```python
from build123d import *

# Parameters (mm, degrees)
BOSS_EXTRUDE1_DEPTH     = 16
SKETCH8_R               = 3.5
CUT_EXTRUDE1_DEPTH      = 16
SKETCH11_R              = 3.5
CUT_EXTRUDE2_DEPTH      = 16
CUT_EXTRUDE3_DEPTH      = 56.172456897
CUT_EXTRUDE3_DEPTH_BACK = 56.172456897
SKETCH12_R              = 3.5
CUT_EXTRUDE4_DEPTH      = 63.497999968
CUT_EXTRUDE4_DEPTH_BACK = 63.497999968
CUT_EXTRUDE5_DEPTH      = 63.497999968
CUT_EXTRUDE5_DEPTH_BACK = 63.497999968


with BuildPart() as part:
    # Sketch3 → Boss-Extrude1 (new body)
    with BuildSketch(Plane.XY):
        Polygon((0, 0), (21, 0), (21, 10), (34, 10), (34, 0), (55, 0), (55, 7), (42, 7), (42, 32), (32, 32), (32, 17), (23, 17), (23, 32), (13, 32), (13, 7), (0, 7), align=None)
    extrude(amount=BOSS_EXTRUDE1_DEPTH)

    # Sketch8 → Cut-Extrude1 (cut)
    with BuildSketch(Plane(origin=(0, 7, 0), x_dir=(1, 0, 0), z_dir=(0, 1, 0))):
        with Locations(Location((6.5, -8, 0), (0, 0, 270))):
            Circle(SKETCH8_R)
    extrude(amount=-CUT_EXTRUDE1_DEPTH, mode=Mode.SUBTRACT)

    # Sketch11 → Cut-Extrude2 (cut)
    with BuildSketch(Plane(origin=(0, 7, 0), x_dir=(1, 0, 0), z_dir=(0, 1, 0))):
        with Locations(Location((48.5, -8, 0), (0, 0, 270))):
            Circle(SKETCH11_R)
    extrude(amount=-CUT_EXTRUDE2_DEPTH, mode=Mode.SUBTRACT)

    # Sketch12 → Cut-Extrude3 (cut, two sides: drawn at the far end of the back side and taken through both)
    with BuildSketch(Plane.ZY.offset(-13).offset(-CUT_EXTRUDE3_DEPTH_BACK)):
        with Locations((8, 24)):
            Circle(SKETCH12_R)
    extrude(amount=CUT_EXTRUDE3_DEPTH + CUT_EXTRUDE3_DEPTH_BACK, mode=Mode.SUBTRACT)

    # Sketch13 → Cut-Extrude4 (cut, two sides: drawn at the far end of the back side and taken through both)
    with BuildSketch(Plane(origin=(0, 7, 0), x_dir=(1, 0, 0), z_dir=(0, 1, 0)).offset(-CUT_EXTRUDE4_DEPTH_BACK)):
        Polygon((6.5, -16), (0, -16), (0, -10), align=None)
    extrude(amount=CUT_EXTRUDE4_DEPTH + CUT_EXTRUDE4_DEPTH_BACK, mode=Mode.SUBTRACT)

    # Sketch14 → Cut-Extrude5 (cut, two sides: drawn at the far end of the back side and taken through both)
    with BuildSketch(Plane(origin=(0, 7, 0), x_dir=(1, 0, 0), z_dir=(0, 1, 0)).offset(-CUT_EXTRUDE5_DEPTH_BACK)):
        Polygon((55, -16), (55, -10), (48.5, -16), align=None)
    extrude(amount=CUT_EXTRUDE5_DEPTH + CUT_EXTRUDE5_DEPTH_BACK, mode=Mode.SUBTRACT)


solid = part.part
```
Can you work these out from the model? Positions are in its coordinate system, mm. A direction names the side the tool comes from. Coordinates: 2 decimals unless noted, no trailing zeros. Order: outer loops, then holes, each group sorted by start corner. A loop starts at its lowest first (then second) coordinate and runs counter-clockwise, first axis right, second up.
1. If we section it at C-C (x = 46): Please give me the cut outline in (y, z).
2. If we section it at D-D (z = 1.25): Please give me the cut outline in (x, y), then the cut area to 3 significant figures.
3. I need wall thicknesses on line 1 (X direction, y = 2, z = 8); line 2 (X direction, y = 19, z = 3.75); line 3 (Y direction, x = 36.25, z = 8). Which ranges of each line are inside material? Lowest first, please.
4. Thinking about a two-plate mould opening in X: for faces 1 (the face through (21, 5, 8)), 2 (the face through (10.4, 0, 7.9)), 3 (the face through (42, 19, 8)), which applies, +X half, -X half, draft (parallel to the pull), parting line (faces both ways), or undercut?
5. If we section it at A-A (z = 8): Give the number of separate pieces and of enclosed holes in the cut face, then the cut area to 3 significant figures.
6. I'm going to push flat-ended pins straight in: pin 1 (5 mm diameter, centred on y = 22.5, z = 4.5, fed in from +X); pin 2 (4 mm diameter, centred on x = 26.5, z = 7, fed in from -Y); pin 3 (8 mm diameter, centred on y = 16, z = 11.5, fed in from -X). Where does each tip first touch, or does it pass through?
7. For faces 4 (the face through (27, 16, 0)), 5 (the face through (4.4, 3.5, 5.2)), 6 (the face through (32, 28, 8)), 7 (the face through (7, 7, 4)), 8 (the face through (49, 7, 4)), which set-ups out of +Z, -Z, +X, -X, +Y, -Y let a thin tool reach every point of the face, with its end or its side?
8. If we section it at B-B (y = 8): Please give me the cut outline in (x, z).
Entries:
1. outline: (0, 0) - (7, 0) - (7, 5.55) - (0, 5.55) - close; (0, 10.45) - (7, 10.45) - (7, 16) - (0, 16) - close
2. outline: (0, 0) - (21, 0) - (21, 10) - (34, 10) - (34, 0) - (55, 0) - (55, 7) - (42, 7) - (42, 32) - (32, 32) - (32, 17) - (23, 17) - (23, 32) - (13, 32) - (13, 7) - (0, 7) - close
2. area: 845 mm2
3. line 1: x = 0 to 3, 10 to 21, 34 to 45, 52 to 55
3. line 2: x = 13 to 23, 32 to 42
3. line 3: y = 0 to 20.5, 27.5 to 32
4. face 1: undercut
4. face 2: draft
4. face 3: +X half
5. separate pieces: 5
5. enclosed holes: 0
5. area: 607 mm2
6. pin 1: stops at x = 42
6. pin 2: stops at y = 10
6. pin 3: stops at x = 13
7. face 4: -Z, +X, -X, +Y, -Y
7. face 5: +Y, -Y
7. face 6: +Z, -Z, +Y
7. face 7: +Z, -Z, -X, +Y
7. face 8: +Z, -Z, +X, +Y
8. outline: (13, 0) - (21, 0) - (21, 16) - (13, 16) - close; (34, 0) - (42, 0) - (42, 16) - (34, 16) - close
